Autodesk Inventor part; units mm, degrees
ref_plane "YZ Plane" through (0, 0, 0) normal (1, 0, 0) x (0, 1, 0)
ref_plane "XZ Plane" through (0, 0, 0) normal (0, 1, 0) x (-1, 0, 0)
ref_plane "XY Plane" through (0, 0, 0) normal (0, 0, 1) x (1, 0, 0)
sketch "Sketch1" plane through (0, 0, 0) normal (0, 0, 1) x (1, 0, 0)
  line L0 (0, 57.15) -> (0, 14.3002)
  line L1 (14.3002, 0) -> (57.15, 0)
  line L2 (57.15, 0) -> (57.15, 4.7752)
  line L3 (57.15, 4.7752) -> (14.3002, 4.7752)
  line L4 (4.7752, 14.3002) -> (4.7752, 57.15)
  line L5 (4.7752, 57.15) -> (0, 57.15)
  arc A0 (4.7752, 14.3002) -> (14.3002, 4.7752) centre (14.3002, 14.3002) ccw
  arc A1 (0, 14.3002) -> (14.3002, 0) centre (14.3002, 14.3002) ccw
  point P0 (0, 0)
  dimension "d0" = 4.7752
  dimension "d1" = 9.525
  dimension "d2" = 14.3002
  dimension "d3" = 57.15
extrude "Extrusion1" add sketch "Sketch1" along normal blind 101.6
hole "Hole1" at (4.7752, 44.45, 88.9) direction (-1, 0, 0) diameter 6.731 end through all
hole "Hole2" at (4.7752, 44.45, 12.7) direction (-1, 0, 0) diameter 6.731 end through all
sketch "Sketch2" plane through (14.3002, 0, 0) normal (0, -1, 0) x (1, 0, 0)
  line L0 (42.8498, 101.6) -> (0, 101.6)
  line L1 (0, 0) -> (42.8498, 0)
  line L2 (42.8498, 0) -> (42.8498, 101.6)
  line L3 (30.1498, 101.6) -> (30.1498, 85.725)
  line L4 (17.4498, 101.6) -> (17.4498, 85.725)
  line L5 (30.1498, 0) -> (30.1498, 15.875)
  line L6 (17.4498, 0) -> (17.4498, 15.875)
  arc A0 (17.4498, 85.725) -> (30.1498, 85.725) centre (23.7998, 85.725) ccw
  arc A1 (30.1498, 15.875) -> (17.4498, 15.875) centre (23.7998, 15.875) ccw
  circle A2 centre (23.7998, 50.8) radius 3.3655
  line L7 (30.1498, 101.6) -> (17.4498, 101.6)
  line L8 (30.1498, 0) -> (17.4498, 0)
  point P0 (-14.3002, 0)
  dimension "d24" = 12.7
  dimension "d25" = 19.05
  dimension "d26" = 15.875
  dimension "d27" = 6.731
  dimension "d28" = 50.8
  dimension "d29" = 19.05
extrude "Extrusion2" cut sketch "Sketch2" against normal blind 101.6
equation "\"d2\" = d1 + d0"
equation "\"d29\" = d25"
properties part number "GE-12073"
Verification items for the finished model (mm, model axes). A direction names the side the tool comes from. Coordinates: 2 decimals unless noted, no trailing zeros. Loops run counter-clockwise (first coordinate to the right, second up) from the corner with the lowest first, then second, coordinate; pieces in that order, holes last. Notation, with made-up numbers: (84, 48) - (123, 48) arc R15 cw to (123, 76) - close; hole circle Ø7 at (62.5, 47). An arc over 180 degrees is marked (long way). Return JSON: item names as keys, results as strings.
1. Section check C-C, the plane z = 88.9. Count the separate pieces of the cut face and the enclosed holes in it, then the cut area to 3 significant figures.
Established:
{"separate pieces": "3", "enclosed holes": "0", "area": "406 mm2"}
2. Thickness scan on L1, parallel to Z at x = 3.15, y = 44.45; L2, parallel to Z at x = 2, y = 44; L3, parallel to X at y = 52.5, z = 41. Record the ranges inside material, lowest first.
Established:
{"L1": "z = 0 to 9.33, 16.07 to 85.53, 92.27 to 101.6", "L2": "z = 0 to 9.36, 16.04 to 85.56, 92.24 to 101.6", "L3": "x = 0 to 4.78"}
3. Tool access check on faces 4 (the flat face through (44.45, 2, 8)), 5 (the flat face through (31.75, 2, 94)), 6 (the flat face through (31, 4.775, 50)). Record the directions out of +Z, -Z, +X, -X, +Y, -Y that give a thin tool (end or side, any length) a straight path to the whole face; none if there is none.
Established:
{"face 4": "-Z, +Y, -Y", "face 5": "+Z, +Y, -Y", "face 6": "+Z, -Z, +X, +Y"}
4. Section check B-B, the plane y = 44.45. Record the boundary of the cut face in (x, z).
Established:
{"outline": "(0, 0) - (4.78, 0) - (4.78, 9.33) - (0, 9.33) - close; (0, 16.07) - (4.78, 16.07) - (4.78, 85.53) - (0, 85.53) - close; (0, 92.27) - (4.78, 92.27) - (4.78, 101.6) - (0, 101.6) - close"}
5. Go/stop test with flat-tipped pins: pin 1 (2.5 mm diameter, centred on y = 3, z = 11.5, fed in from -X); pin 2 (4 mm diameter, centred on x = 38.1, z = 50.8, fed in from +Y); pin 3 (12 mm diameter, centred on x = 41, z = 72.5, fed in from +Y); pin 4 (12 mm diameter, centred on y = 27, z = 67, fed in from -X). Record where each tip stops, or that it passes through.
Established:
{"pin 1": "stops at x = 4.13", "pin 2": "passes through", "pin 3": "stops at y = 4.78", "pin 4": "stops at x = 0"}
6. Mould release check, pull along X, two halves, no side actions. Record for faces 1 (the flat face through (31.75, 2, 8)), 2 (the flat face through (31, 0, 50)), 3 (the flat face through (4.775, 35, 50)): +X half, -X half, draft (parallel to the pull), parting line (faces both ways), or undercut.
Established:
{"face 1": "undercut", "face 2": "draft", "face 3": "+X half"}
7. Section check D-D, the plane y = 33. Record the boundary of the cut face in (x, z).
Established:
{"outline": "(0, 0) - (4.78, 0) - (4.78, 101.6) - (0, 101.6) - close"}
